```python
from build123d import *

# Parameters (mm, degrees)
ESBO_O1_R                = 3.5
ESBO_O1_R_2              = 0.9
ESBO_O1_R_3              = 1.5
ESBO_O1_W                = 5
ESBO_O1_H                = 3
RESSALTO_EXTRUS_O1_DEPTH = 3


with BuildPart() as part:
    # Esboço1 → Ressalto-extrusão1 (new body)
    with BuildSketch(Plane(origin=(0, 0, 0), x_dir=(1, 0, 0), z_dir=(0, 1, 0))):
        with BuildLine():
            Line((-15.5324261, 5.526900759), (-8.701477822, 6.15))
            add(Edge.make_bspline(
                [(8.269723742, 4.259468977), (2.834912713, 6.157347241), (-2.82215339, 6.787527354), (-8.701477822, 6.15)],
                knots=[0.35388944, 0.35388944, 0.35388944, 0.35388944, 1, 1, 1, 1], degree=3))
            ThreePointArc((8.269723742, 4.259468977), (10.737611567, 3.46879666), (13.24315076, 2.807051708))
            add(Edge.make_bspline(
                [(13.243153259, -2.80704963), (25.10877849, 2.12e-06), (13.24315076, 2.807051708)],
                knots=[5.194112275, 5.194112275, 5.194112275, 7.372258742, 7.372258742, 7.372258742], degree=2, weights=[1, 0.463306864, 1]))
            ThreePointArc((13.243153259, -2.80704963), (10.737612779, -3.468795552), (8.269723742, -4.259468977))
            add(Edge.make_bspline(
                [(8.269723742, -4.259468977), (2.834913243, -6.15734876), (-2.822153925, -6.787525817), (-8.701477822, -6.15)],
                knots=[0.35388944, 0.35388944, 0.35388944, 0.35388944, 1, 1, 1, 1], degree=3))
            Line((-8.701477822, -6.15), (-15.5324261, -5.526900759))
            add(Edge.make_bspline(
                [(-91.135478662, -2.939356415), (-85.814709071, -4.330378827), (-60.917561227, -7.97508816), (-35.132432713, -3.48955228), (-15.5324261, -5.526900759)],
                knots=[0.107974898, 0.107974898, 0.107974898, 0.107974898, 0.300967181, 1, 1, 1, 1], degree=3))
            ThreePointArc((-91.135478662, -2.939356415), (-94.330524557, -2.159963767), (-97.549471293, -1.486054958))
            add(Edge.make_bspline(
                [(-97.549471293, 1.486054958), (-105.279311729, 0), (-97.549471293, -1.486054958)],
                knots=[5.195092838, 5.195092838, 5.195092838, 7.371277776, 7.371277776, 7.371277776], degree=2, weights=[1, 0.464175793, 1]))
            ThreePointArc((-97.549471293, 1.486054958), (-94.330524557, 2.159963767), (-91.135478662, 2.939356415))
            add(Edge.make_bspline(
                [(-91.135478662, 2.939356415), (-85.814709071, 4.330378827), (-60.917561227, 7.97508816), (-35.132432713, 3.48955228), (-15.5324261, 5.526900759)],
                knots=[0.107974898, 0.107974898, 0.107974898, 0.107974898, 0.300967181, 1, 1, 1, 1], degree=3))
        make_face()
        Circle(ESBO_O1_R, mode=Mode.SUBTRACT)
        with Locations((10, 0)):
            Circle(ESBO_O1_R_2, mode=Mode.SUBTRACT)
        with Locations((-10, 0)):
            Circle(ESBO_O1_R_2, mode=Mode.SUBTRACT)
        with Locations((-25, 0)):
            Circle(ESBO_O1_R_3, mode=Mode.SUBTRACT)
        with Locations((-75, 0)):
            Circle(ESBO_O1_R_3, mode=Mode.SUBTRACT)
        with Locations((-50, 0)):
            Rectangle(ESBO_O1_W, ESBO_O1_H, mode=Mode.SUBTRACT)
    extrude(amount=RESSALTO_EXTRUS_O1_DEPTH)


solid = part.part
```
The model under review builds one solid part; all positions refer to its coordinate system, in mm. A direction names the side the tool comes from. Round coordinates to 2 decimals unless told otherwise and drop trailing zeros. Use a Markdown table: item, result.
Q1. Mouldability with a two-part tool opening along X and no side actions: class faces 4 (the cylindrical face through (-94.29, 1.48, 2.17)), 5 (the flat face through (-12.165, 1.479, -5.834)), 6 (the cylindrical face through (10.77, 1.48, 3.46)), 7 (the cylindrical face through (-73.57, 1.48, -0.45)) as +X half, -X half, draft (parallel to the pull), parting line (faces both ways), or undercut.
Values:
| item | result |
|---|---|
| face 4 | -X half |
| face 5 | undercut |
| face 6 | +X half |
| face 7 | undercut |
Q2. For line 1 (Z direction, x = 10, y = 1); line 2 (Z direction, x = -10, y = 2.2); line 3 (Z direction, x = -73, y = 1.15), list the stretches that pass through material, from the lowest coordinate up.
Values:
| item | result |
|---|---|
| line 1 | z = -3.69 to -0.9, 0.9 to 3.69 |
| line 2 | z = -6.03 to -0.9, 0.9 to 6.03 |
| line 3 | z = -5.66 to 5.66 |
Q3. Clearance check with a flat-ended pin moving along its axis: P1, Ø1.5, axis at x = -51, y = 1.5, coming from the -Z side. State where the tip first meets the part, or that it passes through.
Values:
| item | result |
|---|---|
| P1 | stops at z = -5.6 |
Q4. Tool access review of faces 1 (the cylindrical face through (10.7, 1.48, -3.48)), 2 (the flat face through (-52.5, 1, 0)), 3 (the flat face through (-12.069, 1.479, 5.843)): name each direction out of +Z, -Z, +X, -X, +Y, -Y from which nothing blocks a thin tool from reaching the whole face with its end or side.
Values:
| item | result |
|---|---|
| face 1 | -Z, +X, +Y, -Y |
| face 2 | +Y, -Y |
| face 3 | +Z, +Y, -Y |
Q5. We need section A-A on y = 1.35. State how many separate pieces and enclosed holes the cut face has, then the cut area to 3 significant figures.
Values:
| item | result |
|---|---|
| separate pieces | 1 |
| enclosed holes | 6 |
| area | 1,070 mm^2 |
